For this review, take the finished solid that the model builds, in its own axes (mm). Coordinates: 2 decimals unless noted, no trailing zeros. Loops run counter-clockwise (first coordinate to the right, second up) from the corner with the lowest first, then second, coordinate; pieces in that order, holes last. Notation, with made-up numbers: M -23.5,-25.75 L -1.5,-25.75 A29 cw -1.5,-5.75 Z; hole C -8,11 d6. An arc over 180 degrees is marked long. Answer as a JSON object with one key per item and string values. Group by question number.
Item 1: Insertion check: pin 1 (21.5 mm diameter, centred on x = -20, y = 31.5, fed in from +Z); pin 2 (3.5 mm diameter, centred on x = 63.58, y = -27.853, fed in from -Z); pin 3 (0.8 mm diameter, centred on x = 28, z = 0.5, fed in from -Y); pin 4 (2.5 mm diameter, centred on x = -70.152, y = -11.65, fed in from -Z). Each pin has a flat end and moves straight along its axis. Give the tip position at first contact, or say it passes through.
Item 2: Mouldability with a two-part tool opening along X and no side actions: class faces 1 (the face through (1, -4.5, -0.038)), 2 (the face through (63.523, 45.703, 0.805)) as +X half, -X half, draft (parallel to the pull), parting line (faces both ways), or undercut.
Item 3: Add section C-C (z = 1.2). State the section outline as (x, y) points (3 decimals), then the cut area to 3 significant figures.
Item 4: Wall thickness on L1, parallel to Y at x = 63.58, z = 1; L2, parallel to X at y = -31.5, z = 1.1; L3, parallel to Z at x = -47.5, y = -31: over which ranges is each line inside the solid? List them lowest first. Write a range as from..to.
Item 5: Add section A-A (y = 23.35). State the section outline as (x, z) points (1 decimal).
from build123d import *

# Parameters (mm, degrees)
SKETCH1_W                = 146.304
SKETCH1_H                = 78.867
BOSS_EXTRUDE1_DEPTH      = 1.5875
BOSS_EXTRUDE2_DEPTH      = 0.0254
BOSS_EXTRUDE2_DEPTH_BACK = 1.6254
SKETCH5_R                = 1.445
CUT_EXTRUDE1_DEPTH       = 2.6254
SKETCH7_W                = 63.5
SKETCH7_H                = 9.144
BOSS_EXTRUDE3_DEPTH      = 1.5875
SKETCH6_R                = 1.397
SKETCH6_R_2              = 1.425015072
CUT_EXTRUDE2_DEPTH       = 2.6254


with BuildPart() as part:
    # Sketch1 → Boss-Extrude1 (new body)
    with BuildSketch(Plane.XY):
        with Locations((0, 9.0805)):
            Rectangle(SKETCH1_W, SKETCH1_H)
    extrude(amount=BOSS_EXTRUDE1_DEPTH)

    # Sketch4 → Boss-Extrude2 (add, two sides)
    with BuildSketch(Plane.XY.offset(1.5875)) as boss_extrude2_sk:
        Polygon((-73.152, 5.08), (73.152, 5.08), (73.152, -5.08), (-23.4823, -5.08), (-23.4823, -30.353), (-33.6423, -30.353), (-33.6423, -5.08), (-73.152, -5.08), align=None)
    extrude(amount=BOSS_EXTRUDE2_DEPTH)
    extrude(boss_extrude2_sk.sketch, amount=-BOSS_EXTRUDE2_DEPTH_BACK)

    # Sketch5 → Cut-Extrude1 (cut, through all)
    with BuildSketch(Plane.XY.offset(1.5875)):
        with Locations((63.58, 47.147)):
            Circle(SKETCH5_R)
        with Locations((63.58, -27.853)):
            Circle(SKETCH5_R)
    extrude(amount=-CUT_EXTRUDE1_DEPTH, mode=Mode.SUBTRACT)

    # Sketch7 → Boss-Extrude3 (add)
    with BuildSketch(Plane.XY.offset(1.5875)):
        with Locations((-41.402, -34.925)):
            Rectangle(SKETCH7_W, SKETCH7_H)
    extrude(amount=-BOSS_EXTRUDE3_DEPTH)

    # Sketch6 → Cut-Extrude2 (cut, through all)
    with BuildSketch(Plane.XY.offset(1.5875)):
        with Locations((-70.152, 23.35)):
            Circle(SKETCH6_R)
        with Locations((-70.152, -11.65)):
            Circle(SKETCH6_R_2)
        with Locations((-60.152, 40.424999886)):
            Circle(SKETCH6_R)
        with Locations((-60.152, -34.575)):
            Circle(SKETCH6_R)
    extrude(amount=-CUT_EXTRUDE2_DEPTH, mode=Mode.SUBTRACT)


solid = part.part
From the geometry:
{
 "1": {"pin 1": "stops at z = 1.59", "pin 2": "stops at z = 0", "pin 3": "stops at y = -30.35", "pin 4": "passes through"},
 "2": {"face 1": "draft", "face 2": "undercut"},
 "3": {"outline": "M -73.152,-39.497 L -9.652,-39.497 L -9.652,-30.353 L 73.152,-30.353 L 73.152,48.514 L 64.048,48.514 A1.445 cw long 63.112,48.514 L -73.152,48.514 Z; hole C -70.152,-11.65 d2.85; hole C -70.152,23.35 d2.794; hole C -60.152,-34.575 d2.794; hole C -60.152,40.425 d2.794; hole C 63.58,-27.853 d2.89", "area": "12,100 mm²"},
 "4": {"L1": "y = -30.35..-29.3, -26.41..45.7", "L2": "x = -73.15..-9.65", "L3": "z = 0..1.59"},
 "5": {"outline": "M -73.2,0 L -71.5,0 L -71.5,1.6 L -73.2,1.6 Z; M -68.8,0 L 73.2,0 L 73.2,1.6 L -68.8,1.6 Z"}
}
